Autodesk Inventor part; units mm, degrees
ref_plane "YZ Plane" through (0, 0, 0) normal (1, 0, 0) x (0, 1, 0)
ref_plane "XZ Plane" through (0, 0, 0) normal (0, 1, 0) x (-1, 0, 0)
ref_plane "XY Plane" through (0, 0, 0) normal (0, 0, 1) x (1, 0, 0)
sketch "Sketch1" plane through (0, 0, 0) normal (0, 0, 1) x (1, 0, 0)
  line L0 (-13, 10) -> (13, 10)
  line L1 (13, 10) -> (13, -10)
  line L2 (13, -10) -> (-13, -10)
  line L3 (-13, -10) -> (-13, 10)
  line L4 (-13, 10) -> (13, -10) construction
  line L5 (13, 10) -> (-13, -10) construction
  line L6 (-16, 13) -> (16, 13)
  line L7 (16, 13) -> (16, -13)
  line L8 (16, -13) -> (-16, -13)
  line L9 (-16, -13) -> (-16, 13)
  line L10 (-16, 13) -> (16, -13) construction
  line L11 (16, 13) -> (-16, -13) construction
  point P0 (0, 0)
  dimension "d0" = 26
  dimension "d1" = 20
  dimension "d2" = 3
  dimension "d3" = 3
extrude "Extrusion1" add sketch "Sketch1" along normal blind 0.508
fillet "Fillet1" radius 1.5875 8 edges at (-13, 10, 0.254) (-13, -10, 0.254) (13, -10, 0.254) (13, 10, 0.254) (16, -13, 0.254) (16, 13, 0.254) (-16, 13, 0.254) (-16, -13, 0.254)
properties part number "Display Bezel" material "Aluminum 6061"
Geometry: final body of the model. Coordinates: model frame, mm. A direction names the side the tool comes from. Give positions to 0.01 mm unless a question says otherwise; leave off trailing zeros. Loops run counter-clockwise (first coordinate to the right, second up) from the corner with the lowest first, then second, coordinate; pieces in that order, holes last. Notation, with made-up numbers: (64.5, 39) - (105.5, 39) arc R24 ccw to (105.5, 64) - close; hole circle Ø1 at (-27, 77). An arc over 180 degrees is marked (long way). Answer as CSV lines item,"result". Start each with the question number.
(1) Mould query, pull axis X, two halves, no side actions, for faces 3 (the face through (-12.52, 9.55, 0.26)), 4 (the face through (15.55, 12.52, 0.26)), 5 (the face through (0, -11, 0.508)). Classes: +X half, -X half, draft (parallel to the pull), parting line (faces both ways), or undercut.
(2) Pin query (flat end, axial travel): P1, Ø1, axis at x = 11, y = -9, coming from the +Z side. Return the tip coordinate at first contact, or that it passes through.
(3) Reachability of faces 1 (the face through (-15.52, 12.55, 0.26)), 2 (the face through (-12.55, -9.52, 0.26)) from +Z, -Z, +X, -X, +Y, -Y: full face, straight path, thin tool, end or side. Return the list, or none.
(4) Section query C-C (z = 0.3). Output: boundary loops of the cut face in (x, y) (1 decimal), and give its area (3 significant figures).
(5) Section query A-A (y = 1.25). Output: boundary loops of the cut face in (x, z).
(6) Section query B-B (x = -1.5). Output: boundary loops of the cut face in (y, z).
(7) Ray query, line 1 along X through (y, z) = (1.5, 0.15); line 2 along Y through (x, z) = (-6.5, 0.1); line 3 along X through (y, z) = (11.5, 0.2). Return the intervals inside material, ascending. Write a range as [from, to].
Worked answers:
1,face 3,"undercut"
1,face 4,"+X half"
1,face 5,"draft"
2,P1,"passes through"
3,face 1,"+Z, -Z, -X, +Y"
3,face 2,"+Z, -Z"
4,outline,"(-16, -11.4) arc R1.6 ccw to (-14.4, -13) - (14.4, -13) arc R1.6 ccw to (16, -11.4) - (16, 11.4) arc R1.6 ccw to (14.4, 13) - (-14.4, 13) arc R1.6 ccw to (-16, 11.4) - close; hole (-13, -8.4) arc R1.6 ccw to (-11.4, -10) - (11.4, -10) arc R1.6 ccw to (13, -8.4) - (13, 8.4) arc R1.6 ccw to (11.4, 10) - (-11.4, 10) arc R1.6 ccw to (-13, 8.4) - close"
4,area,"312 mm^2"
5,outline,"(-16, 0) - (-13, 0) - (-13, 0.51) - (-16, 0.51) - close; (13, 0) - (16, 0) - (16, 0.51) - (13, 0.51) - close"
6,outline,"(-13, 0) - (-10, 0) - (-10, 0.51) - (-13, 0.51) - close; (10, 0) - (13, 0) - (13, 0.51) - (10, 0.51) - close"
7,line 1,"x = [-16, -13], [13, 16]"
7,line 2,"y = [-13, -10], [10, 13]"
7,line 3,"x = [-16, 16]"
